from build123d import *

# Parameters (mm, degrees)
BOSS_EXTRUDE1_DEPTH     = 2.54
CUT_EXTRUDE1_DEPTH      = 1
CUT_EXTRUDE1_DEPTH_BACK = 3.54


with BuildPart() as part:
    # Sketch1 → Boss-Extrude1 (new body)
    with BuildSketch(Plane.XY):
        with BuildLine():
            Line((5.391744354, 14.282870357), (5.391744354, 15.765239208))
            Line((5.391744354, 15.765239208), (4.741317205, 15.765239208))
            Line((4.741317205, 15.765239208), (4.741317205, 17.898035208))
            Line((4.741317205, 17.898035208), (5.066530779, 17.898035208))
            Line((5.066530779, 17.898035208), (5.066530779, 19.876846363))
            Line((5.066530779, 19.876846363), (4.595500514, 19.876846363))
            Line((4.595500514, 19.876846363), (4.595500514, 21.924330523))
            Line((4.595500514, 21.924330523), (5.066530779, 21.924330523))
            Line((5.066530779, 21.924330523), (5.066530779, 25.970641097))
            Line((5.066530779, 25.970641097), (8.827667811, 27.043705429))
            Line((8.827667811, 27.043705429), (15.977546955, 27.444115261))
            Line((15.977546955, 27.444115261), (17.49779469, 27.444115261))
            Line((17.49779469, 27.444115261), (17.49779469, 28.820580801))
            Line((17.49779469, 28.820580801), (17.49779469, 30.468511328))
            Line((17.49779469, 30.468511328), (17.783535415, 33.367238893))
            Line((17.783535415, 33.367238893), (18.335195157, 33.807947262))
            Line((18.335195157, 33.807947262), (27.675822425, 33.807947262))
            Line((27.675822425, 33.807947262), (27.675822425, 37.185188617))
            Line((27.675822425, 37.185188617), (27.675822425, 39.633723234))
            Line((27.675822425, 39.633723234), (28.980773711, 40.33269643))
            Line((28.980773711, 40.33269643), (51.141827963, 41.772000615))
            Line((51.141827963, 41.772000615), (51.141827963, 42.284268418))
            Line((51.141827963, 42.284268418), (52.296667979, 42.902837268))
            Line((52.296667979, 42.902837268), (52.814231672, 42.902837268))
            Line((52.814231672, 42.902837268), (53.607165269, 41.42246617))
            Line((53.607165269, 41.42246617), (53.853833977, 41.42246617))
            Line((53.853833977, 41.42246617), (54.968769782, 42.69106932))
            Line((54.968769782, 42.69106932), (55.239970384, 42.69106932))
            Line((55.239970384, 42.69106932), (55.403969099, 42.384891149))
            Line((55.403969099, 42.384891149), (55.598324769, 42.214078003))
            Line((55.598324769, 42.214078003), (56.003141291, 42.902837268))
            Line((56.003141291, 42.902837268), (57.289041594, 42.902837268))
            Line((57.289041594, 42.902837268), (57.992865427, 42.284268418))
            Line((57.992865427, 42.284268418), (59.425813052, 42.284268418))
            Line((59.425813052, 42.284268418), (70.454348226, 38.609355629))
            Line((70.454348226, 38.609355629), (69.798459804, 36.641012721))
            Line((69.798459804, 36.641012721), (76.698212964, 32.585700195))
            ThreePointArc((76.698212964, 32.585700195), (79.05388987, 30.406820911), (80.286409178, 27.444115261))
            Line((80.286409178, 27.444115261), (80.286409178, 21.776774623))
            Line((80.286409178, 21.776774623), (80.286409178, 16.831637208))
            Line((80.286409178, 16.831637208), (80.795500514, 16.384212686))
            Line((80.795500514, 16.384212686), (79.926633106, 15.395592601))
            Line((79.926633106, 15.395592601), (79.364194198, 15.889902643))
            Line((79.364194198, 15.889902643), (77.747695473, 15.024054782))
            Line((77.747695473, 15.024054782), (77.42948761, 13.121408956))
            Line((77.42948761, 13.121408956), (77.927923916, 13.121408956))
            Line((77.927923916, 13.121408956), (77.927923916, 12.734414773))
            Line((77.927923916, 12.734414773), (77.42948761, 12.734414773))
            Line((77.42948761, 12.734414773), (77.42948761, 12.173202104))
            Line((77.42948761, 12.173202104), (66.096875424, 12.173202104))
            Line((66.096875424, 12.173202104), (66.096875424, 13.121408956))
            Line((66.096875424, 13.121408956), (64.324624891, 13.121408956))
            Line((64.324624891, 13.121408956), (63.852024749, 16.101690785))
            Line((63.852024749, 16.101690785), (61.733497308, 21.0437176))
            Line((61.733497308, 21.0437176), (27.288990511, 21.0437176))
            Line((27.288990511, 21.0437176), (27.288990511, 19.876846363))
            Line((27.288990511, 19.876846363), (26.678188815, 19.54968165))
            Line((26.678188815, 19.54968165), (18.661272623, 19.54968165))
            Line((18.661272623, 19.54968165), (19.000020898, 17.4134882))
            Line((19.000020898, 17.4134882), (15.977546955, 17.4134882))
            Line((15.977546955, 17.4134882), (15.7129382, 19.082147588))
            ThreePointArc((15.7129382, 19.082147588), (15.077518105, 20.548119931), (13.813657174, 21.525611186))
            Line((13.813657174, 21.525611186), (7.510402991, 21.525611186))
            ThreePointArc((7.510402991, 21.525611186), (6.418297754, 20.38537823), (5.919290284, 18.887440786))
            Line((5.919290284, 18.887440786), (5.919290284, 14.282870357))
            Line((5.919290284, 14.282870357), (5.391744354, 14.282870357))
        make_face()
    extrude(amount=BOSS_EXTRUDE1_DEPTH)

    # Sketch2 → Cut-Extrude1 (cut, two sides)
    with BuildSketch(Plane.XY.offset(2.54)) as cut_extrude1_sk:
        with BuildLine():
            Line((19.967423309, 32.496521322), (24.512705526, 32.496521322))
            ThreePointArc((24.512705526, 32.496521322), (26.259153953, 31.800841764), (27.048934293, 30.094881867))
            Line((27.048934293, 30.094881867), (27.151503603, 28.214727135))
            ThreePointArc((27.151503603, 28.214727135), (27.08231277, 28.026246238), (26.897880726, 27.946891081))
            Line((26.897880726, 27.946891081), (19.967423309, 27.946891081))
            Line((19.967423309, 27.946891081), (19.967423309, 32.496521322))
        make_face()
    extrude(amount=CUT_EXTRUDE1_DEPTH, mode=Mode.SUBTRACT)
    extrude(cut_extrude1_sk.sketch, amount=-CUT_EXTRUDE1_DEPTH_BACK, mode=Mode.SUBTRACT)


solid = part.part
Model file for the job. Use its own axes, mm. A direction names the side the tool comes from. Give positions to 0.01 mm unless a question says otherwise; leave off trailing zeros. Order: outer loops, then holes, each group sorted by start corner. A loop starts at its lowest first (then second) coordinate and runs counter-clockwise, first axis right, second up. Notation, with made-up numbers: (-11, -28.75) -> (34, -28.75) arc R22 cw to (34, -18.75) -> close; hole circle Ø5 at (24.25, 2). An arc over 180 degrees is marked (long way). Use CSV: the item, a comma, the result in double quotes.
1. Drill centre lines: line 1 along X through (y, z) = (19, 1.25); line 2 along X through (y, z) = (21, 1.8); line 3 along Y through (x, z) = (13.5, 1). Where is each one in solid material? Low to high. Write a range as from..to.
Outcome:
line 1,"5.07..5.93, 15.73..18.75, 62.61..80.29"
line 2,"4.6..6.89, 14.65..27.29, 61.75..80.29"
line 3,"21.53..27.31"
2. Mould opens along X. For faces 1 (the flat face through (77.59, 14.09, 1.25)), 2 (the cylindrical face through (15.09, 20.53, 1.25)), 3 (the flat face through (72, 12.173, 1)), 4 (the flat face through (64.09, 14.59, 1.25)) say: +X half, -X half, draft (parallel to the pull), parting line (faces both ways), or undercut.
Outcome:
face 1,"+X half"
face 2,"undercut"
face 3,"draft"
face 4,"undercut"
3. Band-saw the part on B-B, the plane x = 10.5. Give the cut face in (y, z).
Outcome:
outline,"(21.53, 0) -> (27.14, 0) -> (27.14, 2.54) -> (21.53, 2.54) -> close"
4. 3-axis set-ups, long thin cutter, end or side, ignore diameter. For faces 5 (the flat face through (45, 21.044, 1)), 6 (the flat face through (5.392, 15, 1)), 7 (the flat face through (19.967, 30, 1)), 8 (the flat face through (23, 33.808, 1)): which of +Z, -Z, +X, -X, +Y, -Y reach the whole face in a straight line?
Outcome:
face 5,"+Z, -Z, -Y"
face 6,"+Z, -Z, -X, -Y"
face 7,"+Z, -Z"
face 8,"+Z, -Z, -X, +Y"
5. Band-saw the part on A-A, the plane x = 69. Give the cut face in (y, z).
Outcome:
outline,"(12.17, 0) -> (39.09, 0) -> (39.09, 2.54) -> (12.17, 2.54) -> close"
6. Drop flat-ended pins along their axis: pin 1 (0.8 mm diameter, centred on x = 10, z = 0.5, fed in from -Y); pin 2 (1.3 mm diameter, centred on x = 18, z = 1.5, fed in from -Y); pin 3 (0.6 mm diameter, centred on y = 20.5, z = 1, fed in from +X); pin 4 (1 mm diameter, centred on x = 31, y = 38, fed in from -Z). Give the stop position or say it passes through.
Outcome:
pin 1,"y = 21.53"
pin 2,"y = 17.41"
pin 3,"x = 80.29"
pin 4,"z = 0"
